```python
from build123d import *

# Parameters (mm, degrees)
F0_R     = 0.685
F1_DEPTH = 1.78
F2_R     = 3.49
F2_R_2   = 2.12
F3_DEPTH = 3.02
F4_R     = 0.58
F5_DEPTH = 1.78


with BuildPart() as f1:
    # F0 (on Top) → F1 (new body)
    with BuildSketch(Plane.XY):
        with BuildLine():
            Line((3.6, 0), (2.4993728816, 16.3928100076))
            ThreePointArc((2.4993728816, 16.3928100076), (0, 18.73), (-2.4993728816, 16.3928100076))
            Line((-2.4993728816, 16.3928100076), (-3.6, 0))
            Line((-3.6, 0), (-2.4993728816, -16.3928100076))
            ThreePointArc((-2.4993728816, -16.3928100076), (0, -18.73), (2.4993728816, -16.3928100076))
            Line((2.4993728816, -16.3928100076), (3.6, 0))
        make_face()
        with Locations((0, -16.045)):
            Circle(F0_R, mode=Mode.SUBTRACT)
        with Locations((0, -12.915)):
            Circle(F0_R, mode=Mode.SUBTRACT)
        with Locations((0, -9.785)):
            Circle(F0_R, mode=Mode.SUBTRACT)
        with Locations((0, -6.655)):
            Circle(F0_R, mode=Mode.SUBTRACT)
        with Locations((0, 6.655)):
            Circle(F0_R, mode=Mode.SUBTRACT)
        with Locations((0, 9.785)):
            Circle(F0_R, mode=Mode.SUBTRACT)
        with Locations((0, 12.915)):
            Circle(F0_R, mode=Mode.SUBTRACT)
        with Locations((0, 16.045)):
            Circle(F0_R, mode=Mode.SUBTRACT)
    extrude(amount=F1_DEPTH)

    # F2 (on face) → F3 (join)
    with BuildSketch(Plane.XY.offset(1.78)):
        Circle(F2_R)
        Circle(F2_R_2, mode=Mode.SUBTRACT)
    extrude(amount=F3_DEPTH)

    # F4 (on face) → F5 (cut, through all)
    with BuildSketch(Plane.XY.offset(1.78)):
        Circle(F4_R)
    extrude(amount=-F5_DEPTH, mode=Mode.SUBTRACT)


solid = f1.part
```
Input: part model. Units: mm. Frame: model coordinates. A direction names the side the tool comes from. Give positions to 0.01 mm unless a question says otherwise; leave off trailing zeros. Loops run counter-clockwise (first coordinate to the right, second up) from the corner with the lowest first, then second, coordinate; pieces in that order, holes last.
1) Reachability of faces 4 (the cylindrical face through (0.05, 18.73, 0.88)), 5 (the cylindrical face through (-0.45, 3.46, 3.27)) from +Z, -Z, +X, -X, +Y, -Y: full face, straight path, thin tool, end or side. Return the list, or none.
A:
face 4: +Z, -Z, +Y
face 5: +Z
2) Contact query for flat-ended pins moving along their axis: pin 1 (1 mm diameter, centred on y = -15, z = 4, fed in from -X); pin 2 (2.5 mm diameter, centred on x = 0, y = 0, fed in from +Z); pin 3 (2 mm diameter, centred on y = -2, z = 2, fed in from -X). Output: stop coordinate, or through.
A:
pin 1: passes through
pin 2: stops at z = 1.78
pin 3: stops at x = -3.53
3) Section query A-A on x = 0. Count the separate pieces of the cut face and the enclosed holes in it, and give its area (3 significant figures).
A:
separate pieces: 10
enclosed holes: 0
area: 53.4 mm2
4) Mould query, pull axis X, two halves, no side actions, for faces 1 (the flat face through (-3.042, 8.311, 0.878)), 2 (the cylindrical face through (-0.05, -18.73, 0.88)), 3 (the cylindrical face through (-0.148, -10.454, 0.878)). Classes: released by +X, released by -X, zero draft, split by the parting line, or undercut.
A:
face 1: released by -X
face 2: split by the parting line
face 3: undercut
5) Line query: L1, parallel to Z at x = -3, y = 7; L2, parallel to Y at x = 0, z = 3.1; L3, parallel to Y at x = 1.75, z = 0.9. Output: solid intervals per line, ascending.
A:
L1: z = 0 to 1.78
L2: y = -3.49 to -2.12, 2.12 to 3.49
L3: y = -18.02 to 18.02
6) Section query C-C on z = 4.1. Return the cut outline in (x, y), and give its area (3 significant figures).
A:
outline: circle Ø6.98 at (0, 0); hole circle Ø4.24 at (0, 0)
area: 24.1 mm2
